Source: three-view drawing plus pictorial views. Frame: mm from the lowest corner of the part. Give positions to 0.01 mm unless a question says otherwise; leave off trailing zeros. Order: outer loops, then holes, each group sorted by start corner. A loop starts at its lowest first (then second) coordinate and runs counter-clockwise, first axis right, second up. Notation, with made-up numbers: M -37.5,38 L -23.5,38 A31 ccw -23.5,70 Z; hole C 22.5,60 d4. An arc over 180 degrees is marked long. Use CSV: the item, a comma, the result in double quotes. Start each with the question number.
1. Section query C-C, the plane z = 2.5. Return the cut outline in (x, y), plus the area to 3 significant figures.
2. Section query B-B, the plane y = 26. Return the cut outline in (x, z), plus the area to 3 significant figures.
3. Mould query, pull axis X, two halves, no side actions, for the marked faces 1 and 2. Classes: released by +X, released by -X, zero draft, split by the parting line, or undercut.
4. Line query: line 1 along Y through (x, z) = (12, 0.55); line 2 along X through (y, z) = (37, 0.9); line 3 along Y through (x, z) = (47, 2.8). Output: solid intervals per line, ascending. Write a range as [from, to].
5. Pin query (flat end, axial travel): P1, Ø1.1, axis at x = 23.5, z = 0.5, coming from the +Y side; P2, Ø12, axis at x = 72.5, y = 9, coming from the -Z side; P3, Ø1.5, axis at x = 14.5, z = 1.5, coming from the -Y side; P4, Ø1.1, axis at x = 25, z = 2.5, coming from the -Y side. Return the tip coordinate at first contact, or that it passes through.
6. Section query A-A, the plane x = 80. Return the cut outline in (y, z).
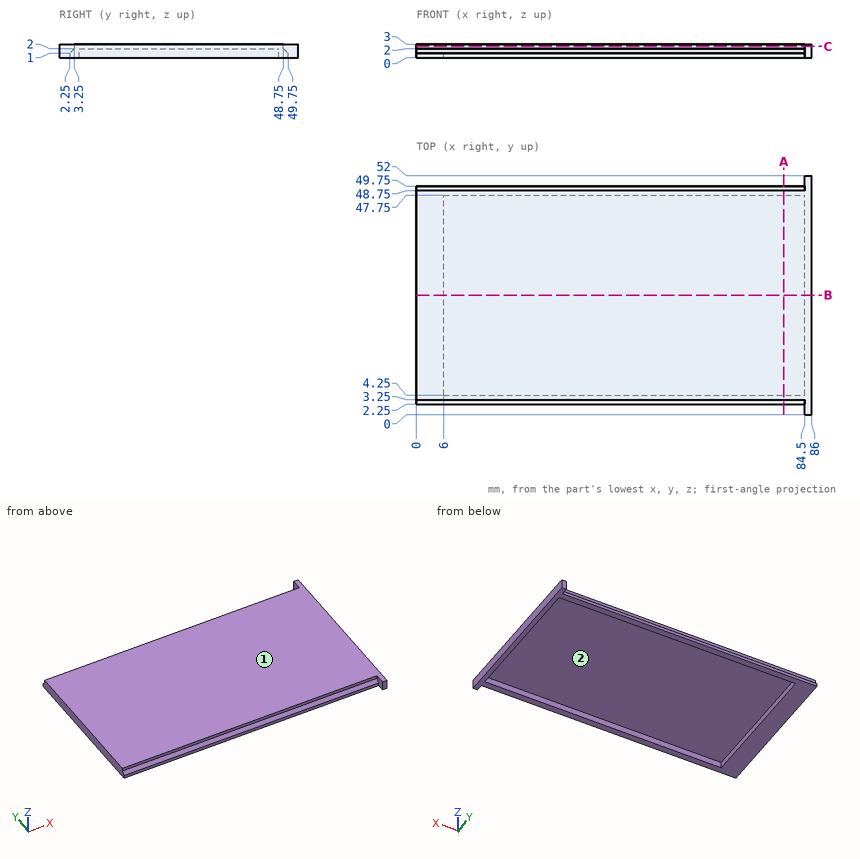
Result set:
1,outline,"M 0,3.25 L 84.5,3.25 L 84.5,0 L 86,0 L 86,52 L 84.5,52 L 84.5,48.75 L 0,48.75 Z"
1,area,"3,920 mm2"
2,outline,"M 0,0 L 6,0 L 6,2 L 84.5,2 L 84.5,0 L 86,0 L 86,3 L 0,3 Z"
2,area,"101 mm2"
3,face 1,"zero draft"
3,face 2,"undercut"
4,line 1,"[2.25, 4.25], [47.75, 49.75]"
4,line 2,"[0, 6], [84.5, 86]"
4,line 3,"[3.25, 48.75]"
5,P1,"y = 49.75"
5,P2,"z = 0"
5,P3,"y = 2.25"
5,P4,"y = 3.2"
6,outline,"M 2.25,0 L 4.25,0 L 4.25,2 L 47.75,2 L 47.75,0 L 49.75,0 L 49.75,1 L 48.75,2 L 48.75,3 L 3.25,3 L 3.25,2 L 2.25,1 Z"
